from build123d import *

# Parameters (mm, degrees)
F0_W      = 200
F0_H      = 460
F1_DEPTH  = 12
F2_W      = 12
F2_H      = 20
F2_W_2    = 20
F2_H_2    = 22
F3_DEPTH  = 25
F4_DEPTH  = 10
F6_W      = 12
F6_H      = 20
F7_DEPTH  = 12
F8_W      = 20
F8_H      = 12
F9_DEPTH  = 25
F11_DEPTH = 25
F12_W     = 5.3429044291
F12_H     = 20
F12_H_2   = 35
F13_DEPTH = 12


# Not quite as in the source:
# - a feature of the source that left no trace in its solid (it failed there, or was rolled back) is left out
# - a feature names something its author has since deleted; it is built from what else it names


with BuildPart() as f1:
    # F0 (on Right) → F1 (new body)
    with BuildSketch(Plane.YZ):
        Polygon((-738, 0), (0, 0), (0, 460), (-70.3818810435, 460), (-172.2238128496, 241.5992724437), (-738, 90), align=None)
        with Locations((100, 230)):
            Rectangle(F0_W, F0_H)
    extrude(amount=F1_DEPTH)

    # F2 (on face) → F3 (cut)
    with BuildSketch(Plane.YZ.offset(12)):
        with Locations((194, 30)):
            Rectangle(F2_W, F2_H)
        with Locations((194, 230)):
            Rectangle(F2_W, F2_H)
        with Locations((194, 420)):
            Rectangle(F2_W, F2_H)
        with Locations((170, 449)):
            Rectangle(F2_W_2, F2_H_2)
        Polygon((-35.0449576251, 460), (-55.0449576251, 460), (-55.0449576251, 450), (-55.0449576251, 438), (-35.0449576251, 438), align=None)
    extrude(amount=-F3_DEPTH, mode=Mode.SUBTRACT)

    # F4 (cut): faces of the model
    f4_faces = [f1.faces().sort_by_distance(p)[0] for p in [
        (6, -62.7134193343, 460),
        (6, 62.4775211875, 460),
        (6, 190, 460),
    ]]
    extrude(f4_faces, amount=-F4_DEPTH, mode=Mode.SUBTRACT)

    # F6 (on face) → F7 (cut)
    with BuildSketch(Plane.XZ.offset(738)):
        with Locations((6, 45)):
            Rectangle(F6_W, F6_H)
    extrude(amount=-F7_DEPTH, mode=Mode.SUBTRACT)

    # F8 (on face) → F9 (cut)
    with BuildSketch(Plane.YZ.offset(12)):
        with Locations((190, 94)):
            Rectangle(F8_W, F8_H)
        Polygon((-70.3818810435, 460), (-75.0449576251, 450), (-70.3818810435, 450), align=None)
    extrude(amount=-F9_DEPTH, mode=Mode.SUBTRACT)

    # F10 (on face) → F11 (cut)
    with BuildSketch(Plane.YZ.offset(12)):
        Polygon((-177.5667172787, 230.14137692), (-172.2238128496, 241.5992724437), (-738, 90), (-738, 79.9737314033), align=None)
    extrude(amount=-F11_DEPTH, mode=Mode.SUBTRACT)

    # F12 (on face) → F13 (join)
    with BuildSketch(Plane.YZ.offset(12)):
        Polygon((-738, 55), (-738, 79.9737314033), (-743.3429044291, 78.5421044763), (-743.3429044291, 55), align=None)
        with Locations((-728.6714522145, 45)):
            Rectangle(F12_W, F12_H)
        with Locations((-740.6714522145, 17.5)):
            Rectangle(F12_W, F12_H_2)
    extrude(amount=-F13_DEPTH)


solid = f1.part
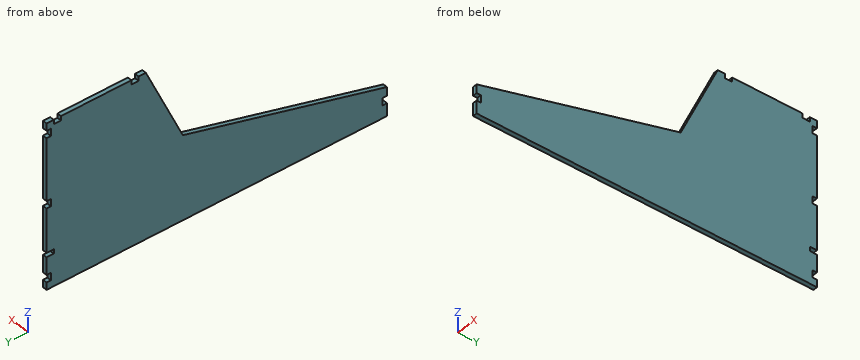
Model file for the job. Use its own axes, mm. Give positions to 0.01 mm unless a question says otherwise; leave off trailing zeros. Order: outer loops, then holes, each group sorted by start corner. A loop starts at its lowest first (then second) coordinate and runs counter-clockwise, first axis right, second up. Notation, with made-up numbers: (-15, 14) - (25, 14) arc R20 ccw to (25, 30) - close; hole circle Ø3 at (38, 20.25). An arc over 180 degrees is marked (long way). One line per item, written item: value.
Item 1: Wall check: line 1 (Y direction, x = 9.25, z = 230.5); line 2 (Z direction, x = 8.5, y = -54.5); line 3 (Y direction, x = 3.25, z = 347). Give the ranges that are in metal, low to high.
Response values:
line 1: -177.4 to 188
line 2: 0 to 438
line 3: -123.07 to 200
Item 2: Pin check, flat tips, straight feed: pin 1 Ø3.5 at (x, z) = (9, 232) entering from +Y; pin 2 Ø3.5 at (x, y) = (9, 170) entering from +Z; pin 3 Ø6 at (x, y) = (6, -737.5) entering from +Z. Stop position of each tip, or through.
Response values:
pin 1: y = 188
pin 2: z = 438
pin 3: z = 80.91
Item 3: Slice it at A-A (z = 264.5). List the corners of the cut face in (x, y), then the cut area to 3 significant figures.
Response values:
outline: (0, -161.55) - (12, -161.55) - (12, 200) - (0, 200) - close
area: 4,340 mm2
Item 4: Slice it at B-B (y = -147). List the corners of the cut face in (x, z).
Response values:
outline: (0, 0) - (12, 0) - (12, 295.69) - (0, 295.69) - close
